The listing builds one solid part. Answer for the finished solid, in the listing's coordinates (mm). Round coordinates to 2 decimals unless told otherwise and drop trailing zeros. Loops run counter-clockwise (first coordinate to the right, second up) from the corner with the lowest first, then second, coordinate; pieces in that order, holes last. Notation, with made-up numbers: (85.25, 75) - (108.25, 75) arc R4 cw to (108.25, 81) - close; hole circle Ø7 at (18, 14). An arc over 180 degrees is marked (long way). Write item = value, one per line. Start each with the question number.
1) Section C-C, the plane z = 0.5 is taken. Determine the outline of the cut face in (x, y).
2) Section D-D, the plane y = -41 is taken. Determine the outline of the cut face in (x, z).
3) Section A-A, the plane y = -22.5 is taken. Determine the outline of the cut face in (x, z).
4) Section B-B, the plane x = -91 is taken. Determine the outline of the cut face in (y, z).
5) Straight lines are drawn through the part: line 1 along X through (y, z) = (-9, 0.45); line 2 along Y through (x, z) = (-107.5, 0.8); line 3 along X through (y, z) = (-29, 0.3). For each, find the intervals that lie inside material, in ascending order.
6) Given pin 1 Ø1 at (y, z) = (-40.5, 1) entering from +X; pin 2 Ø0.6 at (x, z) = (26.5, 1.5) entering from -Y, each flat-ended and moving along its own axis, determine where each tip first touches the part or whether it passes through.
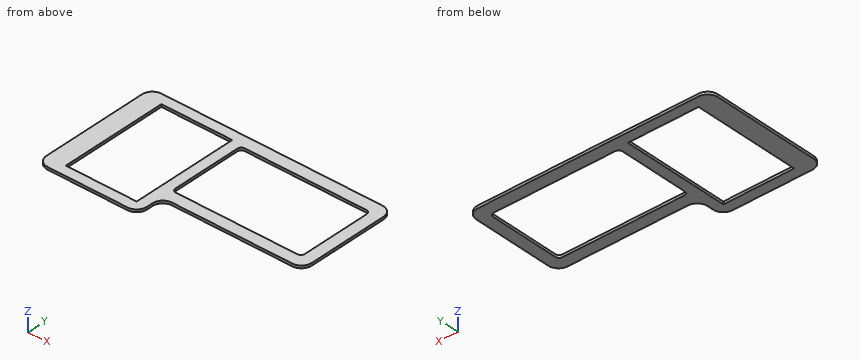
from build123d import *

# Parameters (mm, degrees)
SKETCH1_W          = 54.75
SKETCH1_H          = 83.25
MAIN_EXTRUDE_DEPTH = 2


with BuildPart() as part:
    # Sketch1 → Main extrude (new body)
    with BuildSketch(Plane.XY):
        with BuildLine():
            Line((-50, -51.75), (-50, -47))
            ThreePointArc((-50, -47), (-47.656854249, -41.343145751), (-42, -39))
            Line((-42, -39), (51, -39))
            ThreePointArc((51, -39), (56.656854249, -36.656854249), (59, -31))
            Line((59, -31), (59, 31.5))
            ThreePointArc((59, 31.5), (56.656854249, 37.156854249), (51, 39.5))
            Line((51, 39.5), (-119.75, 39.5))
            ThreePointArc((-119.75, 39.5), (-125.406854249, 37.156854249), (-127.75, 31.5))
            Line((-127.75, 31.5), (-127.75, -51.75))
            ThreePointArc((-127.75, -51.75), (-125.406854249, -57.406854249), (-119.75, -59.75))
            Line((-119.75, -59.75), (-58, -59.75))
            ThreePointArc((-58, -59.75), (-52.343145751, -57.406854249), (-50, -51.75))
        make_face()
        with BuildLine():
            Line((-47, 30), (47, 30))
            ThreePointArc((47, 30), (49.121320344, 29.121320344), (50, 27))
            Line((50, 27), (50, -27))
            ThreePointArc((50, -27), (49.121320344, -29.121320344), (47, -30))
            Line((47, -30), (-47, -30))
            ThreePointArc((-47, -30), (-49.121320344, -29.121320344), (-50, -27))
            Line((-50, -27), (-50, 27))
            ThreePointArc((-50, 27), (-49.121320344, 29.121320344), (-47, 30))
        make_face(mode=Mode.SUBTRACT)
        with Locations((-85.375, -10.125)):
            Rectangle(SKETCH1_W, SKETCH1_H, mode=Mode.SUBTRACT)
    extrude(amount=MAIN_EXTRUDE_DEPTH)


solid = part.part
Geometry check:
q1.outline = (-127.75, -51.75) arc R8 ccw to (-119.75, -59.75) - (-58, -59.75) arc R8 ccw to (-50, -51.75) - (-50, -47) arc R8 cw to (-42, -39) - (51, -39) arc R8 ccw to (59, -31) - (59, 31.5) arc R8 ccw to (51, 39.5) - (-119.75, 39.5) arc R8 ccw to (-127.75, 31.5) - close; hole (-112.75, -51.75) - (-58, -51.75) - (-58, 31.5) - (-112.75, 31.5) - close; hole (-50, -27) arc R3 ccw to (-47, -30) - (47, -30) arc R3 ccw to (50, -27) - (50, 27) arc R3 ccw to (47, 30) - (-47, 30) arc R3 ccw to (-50, 27) - close
q2.outline = (-127.75, 0) - (-112.75, 0) - (-112.75, 2) - (-127.75, 2) - close; (-58, 0) - (-47.29, 0) - (-47.29, 2) - (-58, 2) - close
q3.outline = (-127.75, 0) - (-112.75, 0) - (-112.75, 2) - (-127.75, 2) - close; (-58, 0) - (-50, 0) - (-50, 2) - (-58, 2) - close; (50, 0) - (59, 0) - (59, 2) - (50, 2) - close
q4.outline = (-59.75, 0) - (-51.75, 0) - (-51.75, 2) - (-59.75, 2) - close; (31.5, 0) - (39.5, 0) - (39.5, 2) - (31.5, 2) - close
q5.line_1 = -127.75 to -112.75, -58 to -50, 50 to 59
q5.line_2 = -59.75 to -51.75, 31.5 to 39.5
q5.line_3 = -127.75 to -112.75, -58 to -49.24, 49.24 to 59
q6.pin_1 = -45.87
q6.pin_2 = -39
